Design review of the part built by this model. Coordinates are the model's own, in mm. A direction names the side the tool comes from. Round coordinates to 2 decimals unless told otherwise and drop trailing zeros. Order: outer loops, then holes, each group sorted by start corner. A loop starts at its lowest first (then second) coordinate and runs counter-clockwise, first axis right, second up. Notation, with made-up numbers: M -27.75,34.25 L -7.75,34.25 A37 cw -7.75,72.25 Z; hole C 77,-1 d8. An arc over 180 degrees is marked long. Use a Markdown table: item, result. Add a question column.
(1) For pin 1 (0.8 mm diameter, centred on x = 11.5, y = -1.5, fed in from -Z); pin 2 (3 mm diameter, centred on x = 20.5, y = 3.5, fed in from +Z); pin 3 (2.5 mm diameter, centred on x = 36.75, y = 2.5, fed in from +Z); pin 4 (2 mm diameter, centred on x = 12, z = 4, fed in from +Y), all flat-tipped, find the tip position at first contact; note any pin that passes through.
(2) To check wall thickness, follow probe 1 along Z at (x, y) = (10.5, 5.25); probe 2 along X at (y, z) = (3.5, 2.4); probe 3 along Y at (x, z) = (26.5, 0.6). State the ranges of each line that lie inside material, in increasing order. Write a range as from..to.
(3) Take a section at C-C (z = 3.5). Write out the cut boundary in (x, y).
(4) Machinability: for faces 5 (the face through (11.9, -0.7, 3)), 6 (the face through (12, 4.5, 4)), 7 (the face through (16.051, 2, 4)), which of the approach directions +Z, -Z, +X, -X, +Y, -Y give a long, thin tool a straight path to every point of the face, cutting with its end or side? Answer none if there is none.
(5) Take a section at A-A (y = 2.5). Write out the cut boundary in (x, z).
(6) Take a section at B-B (z = 0.85). Write out the cut boundary in (x, y), then the cut area to 3 significant figures.
(7) Take a section at D-D (y = 11.25). Write out the cut boundary in (x, z).
(8) The part is to be moulded in two halves that separate along Y. For faces 1 (the face through (8.051, 2, 4)), 2 (the face through (35.25, 2.57, 0.99)), 3 (the face through (19, 19, 1)), 4 (the face through (12.18, -0.786, 4.014)), say which applies: released by +Y, released by -Y, zero draft, split by the parting line, or undercut.
```python
from build123d import *

# Parameters (mm, degrees)
F0_W     = 39
F0_H     = 19
F0_R     = 1.5
F1_DEPTH = 2
F2_W     = 8
F2_H     = 4
F3_DEPTH = 4
F6_DEPTH = 2


with BuildPart() as f1:
    # F0 (on Top) → F1 (new body)
    with BuildSketch(Plane.XY):
        with Locations((19.5, 9.5)):
            Rectangle(F0_W, F0_H)
        with Locations((2.7466891247, 2.5)):
            Circle(F0_R, mode=Mode.SUBTRACT)
        with Locations((21.7466891247, 2.5)):
            Circle(F0_R, mode=Mode.SUBTRACT)
        with Locations((36.7466891247, 2.5)):
            Circle(F0_R, mode=Mode.SUBTRACT)
    extrude(amount=F1_DEPTH)

    # F2 (on face) → F3 (join)
    with BuildSketch(Plane.XY.offset(2)):
        with Locations((12.0512238369, 2.5)):
            Rectangle(F2_W, F2_H)
    extrude(amount=F3_DEPTH)

    # F5 (on face) → F6 (join)
    with BuildSketch(Plane.XY.offset(5)):
        Polygon((15.1900717236, 0.915290064), (14.9440382274, 1.3505687319), (9.7206942123, -1.6018332224), (9.9667277085, -2.0371118903), align=None)
    extrude(amount=-F6_DEPTH)


solid = f1.part
```
Verdict:
| question | item | result |
|---|---|---|
| 1 | pin 1 | stops at z = 3 |
| 1 | pin 2 | stops at z = 2 |
| 1 | pin 3 | passes through |
| 1 | pin 4 | stops at y = 4.5 |
| 2 | probe 1 | z = 0..2 |
| 2 | probe 2 | x = 8.05..16.05 |
| 2 | probe 3 | y = 0..19 |
| 3 | outline | M 8.05,0.5 L 13.44,0.5 L 9.72,-1.6 L 9.97,-2.04 L 14.46,0.5 L 16.05,0.5 L 16.05,4.5 L 8.05,4.5 Z |
| 4 | face 5 | +X, -X, -Y |
| 4 | face 6 | +Z, +X, -X, +Y |
| 4 | face 7 | +Z, +X, +Y, -Y |
| 5 | outline | M 0,0 L 1.25,0 L 1.25,2 L 0,2 Z; M 4.25,0 L 20.25,0 L 20.25,2 L 16.05,2 L 16.05,6 L 8.05,6 L 8.05,2 L 4.25,2 Z; M 23.25,0 L 35.25,0 L 35.25,2 L 23.25,2 Z; M 38.25,0 L 39,0 L 39,2 L 38.25,2 Z |
| 6 | outline | M 0,0 L 39,0 L 39,19 L 0,19 Z; hole C 2.75,2.5 d3; hole C 21.75,2.5 d3; hole C 36.75,2.5 d3 |
| 6 | area | 720 mm^2 |
| 7 | outline | M 0,0 L 39,0 L 39,2 L 0,2 Z |
| 8 | face 1 | zero draft |
| 8 | face 2 | undercut |
| 8 | face 3 | released by +Y |
| 8 | face 4 | released by -Y |
